from build123d import *
from OCP.BRepFilletAPI import BRepFilletAPI_MakeChamfer

# Parameters (mm, degrees)
SKETCH1_R           = 8
SKETCH1_W           = 5.5
SKETCH1_H           = 3.7
BOSS_EXTRUDE1_DEPTH = 5
CUT_EXTRUDE1_DEPTH  = 13.369316877
CIRPATTERN1_COUNT   = 6
FILLET1_R           = 10
CHAMFER1_SIZE       = 1
CHAMFER1_SIZE2      = 0.5


with BuildPart() as part:
    # Sketch1 → Boss-Extrude1 (new body)
    with BuildSketch(Plane.XY):
        Circle(SKETCH1_R)
        Rectangle(SKETCH1_W, SKETCH1_H, mode=Mode.SUBTRACT)
    extrude(amount=BOSS_EXTRUDE1_DEPTH)

    # Sketch2 → Cut-Extrude1 (cut, through all)
    with BuildSketch(Plane.XY):
        Polygon((-7.331932906, 22.221764399), (0, 24.952212466), (7.331932906, 22.221764399), (3.798424573, 7.040736522), (3.120998591, 6.924019842), (1.330058439, 5.723612136), (0.501497444, 4.50257488), (-0.501497444, 4.50257488), (-1.330058439, 5.723612136), (-3.120998591, 6.924019842), (-3.798424573, 7.040736522), align=None)
    cut_extrude1 = extrude(amount=CUT_EXTRUDE1_DEPTH, mode=Mode.SUBTRACT)

    # CirPattern1: Cut-Extrude1 ×6 about axis
    cirpattern1_axis = Axis((0, 0, 0), (0, 0, 1))
    for i in range(1, CIRPATTERN1_COUNT):
        add(cut_extrude1.rotate(cirpattern1_axis, i * 360 / CIRPATTERN1_COUNT), mode=Mode.SUBTRACT)

    # Fillet1
    # the kernel refuses this fillet: 10 mm, written as the material it takes off along each edge
    with BuildSketch(Plane(origin=(-1.330058439, -5.723612136, -4.777865205), x_dir=(0.5615014183372642, 0.8274757743917586, 0), z_dir=(0, 0, 1)), Plane(origin=(5.621822731, 1.709941671, -4.777865205), x_dir=(-0.997365750808096, 0.07253660534518461, 0), z_dir=(0, 0, 1)), Plane(origin=(4.291764291, -4.013670465, -4.777865205), x_dir=(-0.43586433247083195, 0.9000123797369435, 0), z_dir=(0, 0, 1)), Plane(origin=(-5.621822731, -1.709941671, -4.777865205), x_dir=(0.997365750808096, -0.07253660534518423, 0), z_dir=(0, 0, 1)), Plane(origin=(-4.291764291, 4.013670465, -4.777865205), x_dir=(0.43586433247083256, -0.900012379736943, 0), z_dir=(0, 0, 1)), Plane(origin=(1.330058439, 5.723612136, -4.777865205), x_dir=(-0.561501418337264, -0.8274757743917588, 0), z_dir=(0, 0, 1))) as fillet1_piece_1:
        with BuildLine():
            CenterArc((1.975419419, 9.987502063), FILLET1_R, 247.992328485, 19.142820558)
            Line((-1.771887917, 0.716165173), (-1.846834064, 0.530738436))
            Line((-1.846834064, 0.530738436), (-0.074946147, -0.185426738))
            Line((-0.074946147, -0.185426738), (0, -0.2))
            ThreePointArc((0, -0.2), (0.737808461, -0.2), (1.465620873, -0.199750041))
            Line((1.465620873, -0.199750041), (1.475616922, 0))
        make_face()
    extrude(amount=14.55573041, mode=Mode.SUBTRACT)
    with BuildSketch(Plane(origin=(5.621822731, -1.709941671, -4.777865205), x_dir=(0.8975096924716217, 0.44099473003596645, 0), z_dir=(0, 0, 1)), Plane(origin=(1.330058439, -5.723612136, -4.777865205), x_dir=(0.8306674853820185, -0.5567688288052, 0), z_dir=(0, 0, 1)), Plane(origin=(-4.291764291, -4.013670465, -4.777865205), x_dir=(-0.06684220708960342, -0.9977635588411669, 0), z_dir=(0, 0, 1)), Plane(origin=(-5.621822731, 1.709941671, -4.777865205), x_dir=(-0.8975096924716216, -0.44099473003596684, 0), z_dir=(0, 0, 1)), Plane(origin=(4.291764291, 4.013670465, -4.777865205), x_dir=(0.06684220708960296, 0.9977635588411669, 0), z_dir=(0, 0, 1)), Plane(origin=(-1.330058439, 5.723612136, -4.777865205), x_dir=(-0.8306674853820185, 0.5567688288052001, 0), z_dir=(0, 0, 1))) as fillet1_piece_2:
        with BuildLine():
            CenterArc((1.911146082, 10), FILLET1_R, 250.857179442, 19.142820558)
            Line((-1.368094161, 0.552959012), (-1.433678966, 0.364018192))
            ThreePointArc((-1.433678966, 0.364018192), (-0.758993227, 0.091052768), (-0.074946147, -0.185426738))
            Line((-0.074946147, -0.185426738), (0, -0.2))
            Line((0, -0.2), (1.911146082, -0.2))
            Line((1.911146082, -0.2), (1.911146082, 0))
        make_face()
    extrude(amount=14.55573041, mode=Mode.SUBTRACT)

    # Chamfer1: one chamfer whose edges measure the first distance from different faces: ONE call of the kernel's chamfer builder (chamfer() names one face for all edges)
    chamfer1_edges_1 = [part.edges().sort_by_distance(p)[0] for p in [
        (-2.75, 0, 0),
    ]]
    chamfer1_side_1 = [part.faces().sort_by_distance(p)[0] for p in [
        (-2.75, 0, 2.5),
    ]]
    chamfer1_edges_2 = [part.edges().sort_by_distance(p)[0] for p in [
        (0, -1.85, 0),
    ]]
    chamfer1_side_2 = [part.faces().sort_by_distance(p)[0] for p in [
        (0, -1.85, 2.5),
    ]]
    chamfer1_edges_3 = [part.edges().sort_by_distance(p)[0] for p in [
        (2.75, 0, 0),
    ]]
    chamfer1_side_3 = [part.faces().sort_by_distance(p)[0] for p in [
        (2.75, 0, 2.5),
    ]]
    chamfer1_edges_4 = [part.edges().sort_by_distance(p)[0] for p in [
        (0, 1.85, 0),
    ]]
    chamfer1_side_4 = [part.faces().sort_by_distance(p)[0] for p in [
        (0, 1.85, 2.5),
    ]]
    chamfer1 = BRepFilletAPI_MakeChamfer(part.part.solid().wrapped)
    for e in chamfer1_edges_1:
        chamfer1.Add(CHAMFER1_SIZE, CHAMFER1_SIZE2, e.wrapped, chamfer1_side_1[0].wrapped)  # the first distance lies on this face
    for e in chamfer1_edges_2:
        chamfer1.Add(CHAMFER1_SIZE, CHAMFER1_SIZE2, e.wrapped, chamfer1_side_2[0].wrapped)  # the first distance lies on this face
    for e in chamfer1_edges_3:
        chamfer1.Add(CHAMFER1_SIZE, CHAMFER1_SIZE2, e.wrapped, chamfer1_side_3[0].wrapped)  # the first distance lies on this face
    for e in chamfer1_edges_4:
        chamfer1.Add(CHAMFER1_SIZE, CHAMFER1_SIZE2, e.wrapped, chamfer1_side_4[0].wrapped)  # the first distance lies on this face
    add(Compound.cast(chamfer1.Shape()), mode=Mode.REPLACE)


solid = part.part
Work out the finished part from the listing and answer in its coordinate system (mm). A direction names the side the tool comes from. Give positions to 0.01 mm unless a question says otherwise; leave off trailing zeros. Order: outer loops, then holes, each group sorted by start corner. A loop starts at its lowest first (then second) coordinate and runs counter-clockwise, first axis right, second up. Notation, with made-up numbers: (62.25, 3) -> (117.25, 3) arc R29 ccw to (117.25, 29) -> close; hole circle Ø3 at (84.5, 88.5). An arc over 180 degrees is marked (long way). Answer as a JSON object with one key per item and string values. Group by question number.
1. Section C-C on x = 1.75 is taken. Determine the outline of the cut face in (y, z), plus the area to 3 significant figures.
2. Section A-A on y = 5 is taken. Determine the outline of the cut face in (x, z).
3. Consider line 1 along X through (y, z) = (0, 3.9); line 2 along Y through (x, z) = (2.5, 3.1); line 3 along X through (y, z) = (-4.75, 0.95). Determine where each line is inside the solid, lowest interval first. Write a range as [from, to].
4. A tool of negligible diameter and unlimited length cuts with its end or side. For faces 1 (the flat face through (2.75, 0, 3)), 2 (the cylindrical face through (-1.63, -5.76, 2.47)), 3 (the cylindrical face through (4.175, -4.294, 2.465)), 4 (the cylindrical face through (-4.175, 4.294, 2.465)), from which of +Z, -Z, +X, -X, +Y, -Y can it reach the whole face along a straight path? Write none if from no direction.
5. Flat-ended cylindrical pins translate along their axes: pin 1 Ø1.2 at (x, z) = (1, 2.5) entering from +Y; pin 2 Ø1 at (y, z) = (-4, 4) entering from -X; pin 3 Ø1.1 at (x, z) = (0, 1.5) entering from +Y. Find the tip coordinate at first contact, or state that the pin passes through.
6. Section B-B on x = -2.25 is taken. Determine the outline of the cut face in (y, z), plus the area to 3 significant figures.
7. Section D-D on x = -4.75 is taken. Determine the outline of the cut face in (y, z).
8. The mould has two halves that part along X. Classify faces 5 (the cylindrical face through (-4.164, -4.248, 2.465)), 6 (the flat face through (0, 4.503, 2)), 7 (the cylindrical face through (5.806, 1.469, 2.465)): released by +X, released by -X, zero draft, split by the parting line, or undercut.
Result sheet:
{
 "1": {"outline": "(-5.87, 0) -> (-2.35, 0) -> (-1.85, 1) -> (-1.85, 5) -> (-5.87, 5) -> close; (1.85, 1) -> (2.35, 0) -> (5.87, 0) -> (5.87, 5) -> (1.85, 5) -> close", "area": "39.7 mm^2"},
 "2": {"outline": "(-4.31, 0) -> (-0.9, 0) -> (-0.9, 5) -> (-4.31, 5) -> close; (0.9, 0) -> (4.31, 0) -> (4.31, 5) -> (0.9, 5) -> close"},
 "3": {"line 1": "x = [-8, -2.75], [2.75, 8]", "line 2": "y = [-6.49, -1.85], [1.85, 6.49]", "line 3": "x = [-4.27, -0.69], [0.69, 4.27]"},
 "4": {"face 1": "+Z, -Z", "face 2": "+Z, -Z, -Y", "face 3": "+Z, -Z, +X", "face 4": "+Z, -Z, -X"},
 "5": {"pin 1": "stops at y = 5.73", "pin 2": "stops at x = -4.22", "pin 3": "stops at y = 4.57"},
 "6": {"outline": "(-6.3, 0) -> (-2.35, 0) -> (-1.85, 1) -> (-1.85, 5) -> (-6.3, 5) -> close; (1.85, 1) -> (2.35, 0) -> (6.3, 0) -> (6.3, 5) -> (1.85, 5) -> close", "area": "44.0 mm^2"},
 "7": {"outline": "(-1.72, 0) -> (1.72, 0) -> (1.72, 5) -> (-1.72, 5) -> close"},
 "8": {"face 5": "released by -X", "face 6": "undercut", "face 7": "released by +X"}
}
